```python
from build123d import *

# Parameters (mm, degrees)
BOSS_EXTRUDE1_DEPTH = 20
SKETCH3_R           = 1.75
CUT_EXTRUDE1_DEPTH  = 46.641220998
SKETCH4_R           = 3
SKETCH4_R_2         = 1.75
SKETCH4_R_3         = 4
CUT_EXTRUDE2_DEPTH  = 45.250661625
FILLET2_R           = 2.5
FILLET3_R           = 0.3


with BuildPart() as part:
    # Sketch2 → Boss-Extrude1 (new body)
    with BuildSketch(Plane.XY):
        Polygon((0, 0), (0, 15), (-5, 15), (-5, 31.814648696), (0, 31.814648696), (10, 38.185351304), (10, 0), align=None)
    extrude(amount=BOSS_EXTRUDE1_DEPTH)

    # Sketch3 → Cut-Extrude1 (cut, through all)
    with BuildSketch(Plane(origin=(10, 0, 0), x_dir=(0, 0, -1), z_dir=(1, 0, 0))):
        with Locations((-15, 7.5)):
            Circle(SKETCH3_R)
        with Locations((-5, 7.5)):
            Circle(SKETCH3_R)
    extrude(amount=-CUT_EXTRUDE1_DEPTH, mode=Mode.SUBTRACT)

    # Sketch4 → Cut-Extrude2 (cut, through all)
    with BuildSketch(Plane.XY.offset(20)):
        with Locations((5, 33.71)):
            Circle(SKETCH4_R)
        with Locations((5, 25)):
            Circle(SKETCH4_R_2)
        with Locations((-7.5, 25)):
            Circle(SKETCH4_R_3)
        with Locations((5, 15)):
            Circle(SKETCH4_R_2)
    extrude(amount=-CUT_EXTRUDE2_DEPTH, mode=Mode.SUBTRACT)

    # Fillet2
    # the kernel refuses this fillet: 2.5 mm, written as the material it takes off along each edge
    with BuildSketch(Plane(origin=(10, 38.185351304, -11.119166033), x_dir=(0, -1, 0), z_dir=(0, 0, 1))) as fillet2_piece_1:
        with BuildLine():
            CenterArc((4.447666413, -2.5), FILLET2_R, 90, 106.897304497)
            Line((2.055598265, -3.226642949), (2.007756902, -3.241175808))
            ThreePointArc((2.007756902, -3.241175808), (0.98562956, -1.640186455), (-0.042169572, -0.02686498))
            Line((-0.042169572, -0.02686498), (0, 0.05))
            Line((0, 0.05), (4.447666413, 0.05))
            Line((4.447666413, 0.05), (4.447666413, 0))
        make_face()
    extrude(amount=42.238332065, mode=Mode.SUBTRACT)
    with BuildSketch(Plane(origin=(-5, 31.814648696, -6.25), x_dir=(1, 0, 0), z_dir=(0, 0, 1))) as fillet2_piece_2:
        with BuildLine():
            CenterArc((FILLET2_R, -FILLET2_R), FILLET2_R, 90, 90)
            Line((0, -FILLET2_R), (-FILLET2_R * 0.02, -FILLET2_R))
            Line((-FILLET2_R * 0.02, -FILLET2_R), (-FILLET2_R * 0.02, FILLET2_R * 0.02))
            Line((-FILLET2_R * 0.02, FILLET2_R * 0.02), (FILLET2_R, FILLET2_R * 0.02))
            Line((FILLET2_R, FILLET2_R * 0.02), (FILLET2_R, 0))
        make_face()
    extrude(amount=32.5, mode=Mode.SUBTRACT)

    # Fillet3
    fillet3_edges = [part.edges().sort_by_distance(p)[0] for p in [
        (2.057505904, 33.125424519, 10),
    ]]
    fillet(fillet3_edges, radius=FILLET3_R)


solid = part.part
```
Could you check a few things on this model? Use its own coordinates, in mm. A direction names the side the tool comes from. Round coordinates to 2 decimals unless told otherwise and drop trailing zeros. Write each loop counter-clockwise with the first axis right and the second up, starting at its lowest first coordinate (ties: lowest second). Pieces come first, ordered by that corner, then holes.
(1) Suppose I cut it at C-C on y = 7.5. Write out the boundary of the cut face in (x, z).
Findings below:
outline: (0, 0) - (10, 0) - (10, 3.25) - (0, 3.25) - close; (0, 6.75) - (10, 6.75) - (10, 13.25) - (0, 13.25) - close; (0, 16.75) - (10, 16.75) - (10, 20) - (0, 20) - close
(2) Suppose I cut it at D-D on y = 25. Write out the boundary of the cut face in (x, z).
Findings below:
outline: (-3.5, 0) - (3.25, 0) - (3.25, 20) - (-3.5, 20) - close; (6.75, 0) - (10, 0) - (10, 20) - (6.75, 20) - close
(3) If I drill on probe 1 along Y at (x, z) = (5, 15); probe 2 along Y at (x, z) = (5, 9.75); probe 3 along Y at (x, z) = (6, 6), over which ranges is the centre line in solid material (lowest first)?
Findings below:
probe 1: y = 0 to 5.75, 9.25 to 13.25, 16.75 to 23.25, 26.75 to 30.71
probe 2: y = 0 to 13.25, 16.75 to 23.25, 26.75 to 30.71
probe 3: y = 0 to 6.06, 8.94 to 13.56, 16.44 to 23.56, 26.44 to 30.88
(4) Which directions (+Z, -Z, +X, -X, +Y, -Y) give clear straight access to the entire face, cutting with the end or side of a thin tool? Please do faces 4 (the face through (-1, 31.815, 10)), 5 (the face through (5.07, 5.79, 5.38)), 6 (the face through (0, 7, 10)).
Findings below:
face 4: +Z, -Z, -X, +Y
face 5: +X, -X
face 6: +Z, -Z, -X, -Y
(5) Thinking about a two-plate mould opening in Z: for faces 1 (the face through (4, 18, 20)), 2 (the face through (-5, 18, 10)), 3 (the face through (5.07, 6.83, 13.383)), which applies, +Z half, -Z half, draft (parallel to the pull), parting line (faces both ways), or undercut?
Findings below:
face 1: +Z half
face 2: draft
face 3: undercut
(6) For pin 1 (4 mm diameter, centred on y = 7.5, z = 5, fed in from -X); pin 2 (4.5 mm diameter, centred on x = 5, y = 15, fed in from +Z); pin 3 (0.8 mm diameter, centred on x = -1.5, z = 9.5, fed in from +Y); pin 4 (2 mm diameter, centred on x = -2.5, z = 11.5, fed in from -Y), each with a flat end and sliding along its axis, tell me the tip position at first contact or that it passes through.
Findings below:
pin 1: stops at x = 0
pin 2: stops at z = 20
pin 3: stops at y = 31.81
pin 4: stops at y = 15
(7) Suppose I cut it at A-A on z = 5. Write out the boundary of the cut face in (x, y), and give its area (3 significant figures).
Findings below:
outline: (-5, 15) - (0, 15) - (0, 9.25) - (10, 9.25) - (10, 33.74) arc R2.5 ccw to (6.77, 36.13) arc R3 cw (long way) to (2.16, 32.75) arc R0.3 ccw to (1.71, 32.91) - (0, 31.81) - (-2.5, 31.81) arc R2.5 ccw to (-5, 29.31) - (-5, 28.12) arc R4 cw to (-5, 21.88) - close; (0, 0) - (10, 0) - (10, 5.75) - (0, 5.75) - close; hole circle Ø3.5 at (5, 15); hole circle Ø3.5 at (5, 25)
area: 347 mm2
(8) Suppose I cut it at B-B on x = 5. Write out the boundary of the cut face in (y, z), and give its area (3 significant figures).
Findings below:
outline: (0, 0) - (13.25, 0) - (13.25, 20) - (0, 20) - close; (16.75, 0) - (23.25, 0) - (23.25, 20) - (16.75, 20) - close; (26.75, 0) - (30.71, 0) - (30.71, 20) - (26.75, 20) - close; hole circle Ø3.5 at (7.5, 5); hole circle Ø3.5 at (7.5, 15)
area: 455 mm2
